from build123d import *

# Parameters (mm, degrees)
SKETCH1_R               = 8.895
BOSS_EXTRUDE1_DEPTH     = 25
CUT_EXTRUDE1_DEPTH      = 12.5
SKETCH3_R               = 1.984375
CUT_EXTRUDE2_DEPTH      = 9.895
CUT_EXTRUDE2_DEPTH_BACK = 9.895
CHAMFER1_SIZE           = 0.8


with BuildPart() as part:
    # Sketch1 → Boss-Extrude1 (new body)
    with BuildSketch(Plane(origin=(0, 0, 0), x_dir=(1, 0, 0), z_dir=(0, 1, 0))):
        Circle(SKETCH1_R)
    extrude(amount=-BOSS_EXTRUDE1_DEPTH)

    # Sketch2 → Cut-Extrude1 (cut)
    with BuildSketch(Plane.XZ.offset(25)):
        with BuildLine():
            Line((-6.83125, 1.984375), (-6.83125, -1.984375))
            Line((-6.83125, -1.984375), (-8.670829306, -1.984375))
            ThreePointArc((-8.670829306, -1.984375), (-8.895, 0), (-8.670829306, 1.984375))
            Line((-8.670829306, 1.984375), (-6.83125, 1.984375))
        make_face()
    cut_extrude1 = extrude(amount=-CUT_EXTRUDE1_DEPTH, mode=Mode.SUBTRACT)

    # Mirror1: Cut-Extrude1 across plane
    add(cut_extrude1.mirror(Plane(origin=(0, 0, 0), x_dir=(0, 0, 1), z_dir=(1, 0, 0))), mode=Mode.SUBTRACT)

    # Sketch3 → Cut-Extrude2 (cut, two sides)
    with BuildSketch(Plane(origin=(0, 0, 0), x_dir=(0, 0, -1), z_dir=(1, 0, 0))) as cut_extrude2_sk:
        with Locations((0, -12.5)):
            Circle(SKETCH3_R)
    extrude(amount=CUT_EXTRUDE2_DEPTH, mode=Mode.SUBTRACT)
    extrude(cut_extrude2_sk.sketch, amount=-CUT_EXTRUDE2_DEPTH_BACK, mode=Mode.SUBTRACT)

    # Sketch4 → Revolve1 (revolve)
    with BuildSketch(Plane(origin=(0, 0, 0), x_dir=(0, 0, -1), z_dir=(1, 0, 0))):
        with BuildLine():
            Line((9.75, 0), (0, 0))
            Line((0, 0), (0, 76.2))
            add(Edge.make_bspline(
                [(0, 76.2), (0.00748237, 76.196303135), (0.026185272, 76.182931832), (0.048569166, 76.155115052), (0.079016608, 76.11449371), (0.114693992, 76.05782259), (0.160958307, 75.977185044), (0.230182007, 75.841272979), (0.337513198, 75.60317482), (0.508759946, 75.169356672), (0.780720305, 74.373974862), (1.175421329, 73.034171439), (1.784765583, 70.644843338), (2.516344519, 67.293069495), (3.309621674, 63.159543132), (4.115536163, 58.4526801), (4.851127077, 53.734453502), (5.69775641, 47.825772453), (6.460335776, 41.90557874), (7.150044053, 35.976499089), (7.770075125, 30.039829718), (8.224479166, 25.286332313), (8.636093389, 20.528933412), (8.956570125, 16.362955309), (9.199825181, 12.789854007), (9.378943901, 9.810771277), (9.506266384, 7.426602256), (9.610457186, 5.15707962), (9.681192933, 3.242776152), (9.725789572, 1.68405962), (9.742877783, 0.721793084), (9.75, 0.240606643), (9.75, 0)],
                knots=[0, 0, 0, 0, 0, 0.000432339, 0.001198718, 0.001819119, 0.002652992, 0.00389752, 0.006030224, 0.009732147, 0.016211386, 0.028104504, 0.049663776, 0.082235971, 0.144220966, 0.206205912, 0.268191171, 0.33017619, 0.392161358, 0.51613157, 0.578116694, 0.64010179, 0.702086952, 0.764072089, 0.826057153, 0.857049723, 0.888042292, 0.919034838, 0.950027383, 0.975013692, 0.987506846, 1, 1, 1, 1, 1], degree=4))
        make_face()
    revolve(axis=Axis((0, 0, 0), (0, 1, 0)))

    # Chamfer1
    chamfer1_edges = [part.edges().sort_by_distance(p)[0] for p in [
        (-8.895, 0, 0),
    ]]
    chamfer(chamfer1_edges, length=CHAMFER1_SIZE)


solid = part.part
The model under review builds one solid part; all positions refer to its coordinate system, in mm. A direction names the side the tool comes from. Round coordinates to 2 decimals unless told otherwise and drop trailing zeros. Order: outer loops, then holes, each group sorted by start corner. A loop starts at its lowest first (then second) coordinate and runs counter-clockwise, first axis right, second up. Notation, with made-up numbers: (2, 24) - (46, 24) arc R30 cw to (46, 49) - close; hole circle Ø3 at (-29, 67.25). An arc over 180 degrees is marked (long way). Use one line per item in the form item = value.
Q1. Add section A-A on y = -3. Give the boundary of the cut face in (x, z) (3 decimals), then the cut area to 3 significant figures.
Response values:
outline = circle Ø17.79 at (0, 0)
area = 249 mm^2
Q2. Clearance check with flat-ended pins moving along their axes: P1, Ø0.9, axis at x = -8, y = -17, coming from the +Z side; P2, Ø0.6, axis at x = -8, y = -21, coming from the -Z side; P3, Ø1.5, axis at x = 7.5, y = -20, coming from the -Z side. State where each tip first meets the part, or that it passes through.
Response values:
P1 = 4.7
P2 = -4.45
P3 = -5.79
Q3. Tool access review of faces 1 (the flat face through (8, -19, 1.984)), 2 (the cylindrical face through (8.484, -12.731, -2.672)), 3 (the flat face through (-8, -19, 1.984)): name each direction out of +Z, -Z, +X, -X, +Y, -Y from which nothing blocks a thin tool from reaching the whole face with its end or side.
Response values:
face_1 = +X, -Y
face_2 = -Y
face_3 = -X, -Y
Q4. To check wall thickness, follow line 1 (Z direction, x = -2, y = -12.5); line 2 (Z direction, x = -0.5, y = -6.5); line 3 (Z direction, x = -6.25, y = -19). State the ranges of each line that lie inside material, in increasing order.
Response values:
line_1 = -8.67 to -1.98, 1.98 to 8.67
line_2 = -8.88 to 8.88
line_3 = -6.33 to 6.33
